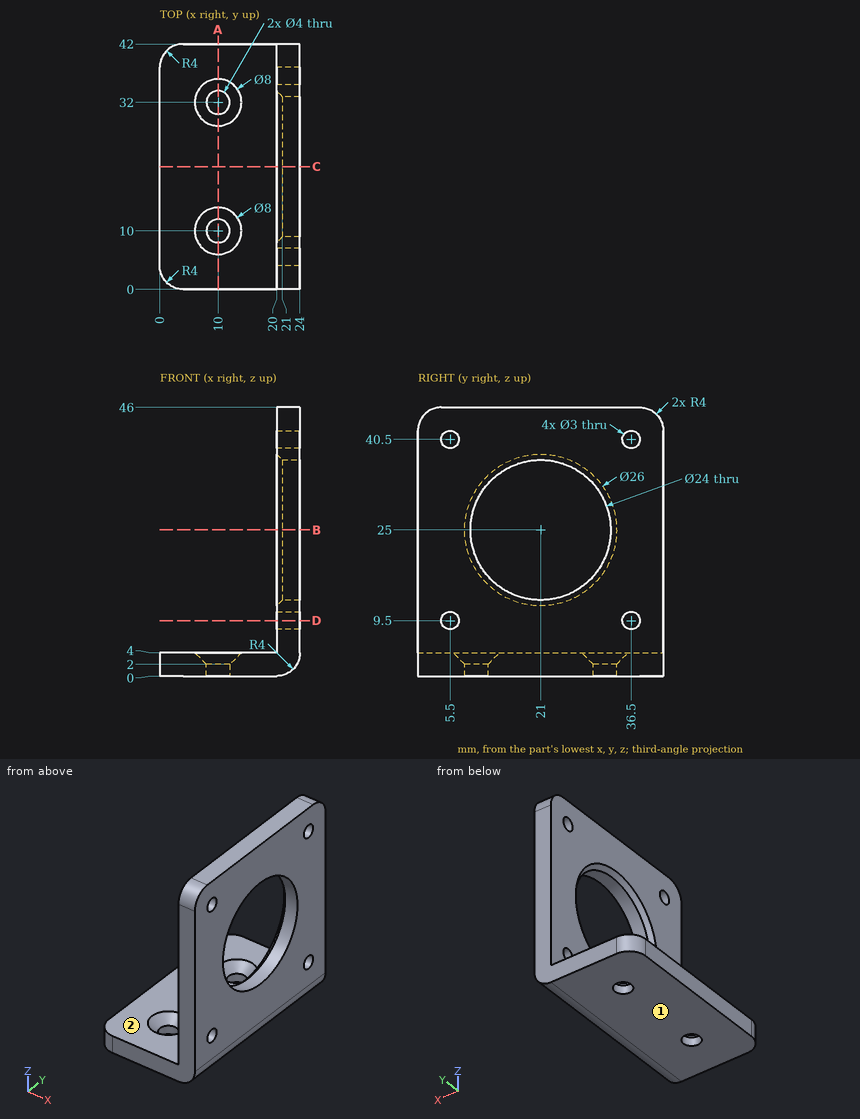
Study the drawing (mm; zero at the part's minimum x, y, z) and answer. A direction names the side the tool comes from. Round coordinates to 2 decimals unless told otherwise and drop trailing zeros. Write each loop counter-clockwise with the first axis right and the second up, starting at its lowest first coordinate (ties: lowest second). Pieces come first, ordered by that corner, then holes.
1) Straight lines are drawn through the part: line 1 (Y direction, x = 22, z = 9.5); line 2 (Y direction, x = 10, z = 1.45); line 3 (Y direction, x = 21.7, z = 25). For each, find the intervals that lie inside material, in ascending order.
2) A cutting plane is placed at B-B (z = 25). Give the vertices of the cut face in (x, y), plus the area to 3 significant figures.
3) Given pin 1 Ø4 at (y, z) = (5.5, 9.5) entering from -X; pin 2 Ø6 at (x, z) = (16, 16) entering from +Y; pin 3 Ø4 at (y, z) = (36.5, 9.5) entering from +X; pin 4 Ø5 at (x, y) = (8.5, 25.5) entering from +Z, each flat-ended and moving along its own axis, determine where each tip first touches the part or whether it passes through.
4) A tool of negligible diameter and unlimited length cuts with its end or side. For the marked faces 1 and 2, from which of +Z, -Z, +X, -X, +Y, -Y can it reach the whole face along a straight path? Write none if from no direction.
5) A cutting plane is placed at C-C (y = 21). Give the vertices of the cut face in (x, z).
6) A cutting plane is placed at D-D (z = 9.5). Give the vertices of the cut face in (x, y).
7) A cutting plane is placed at A-A (x = 10). Give the vertices of the cut face in (y, z), plus the area to 3 significant figures.
Completed:
1. line 1: y = 0 to 4, 7 to 35, 38 to 42
1. line 2: y = 0 to 8, 12 to 30, 34 to 42
1. line 3: y = 0 to 9, 33 to 42
2. outline: (20, 0) - (24, 0) - (24, 9) - (21, 9) - (20, 8) - close; (20, 34) - (21, 33) - (24, 33) - (24, 42) - (20, 42) - close
2. area: 71.0 mm2
3. pin 1: stops at x = 20
3. pin 2: passes through
3. pin 3: stops at x = 24
3. pin 4: stops at z = 4
4. face 1: -Z, +X, -X, +Y, -Y
4. face 2: +Z, -X, +Y, -Y
5. outline: (0, 0) - (20, 0) arc R4 ccw to (24, 4) - (24, 13) - (21, 13) - (20, 12) - (20, 4) - (0, 4) - close; (20, 38) - (21, 37) - (24, 37) - (24, 46) - (20, 46) - close
6. outline: (20, 0) - (24, 0) - (24, 4) - (20, 4) - close; (20, 7) - (24, 7) - (24, 35) - (20, 35) - close; (20, 38) - (24, 38) - (24, 42) - (20, 42) - close
7. outline: (0, 0) - (8, 0) - (8, 2) - (6, 4) - (0, 4) - close; (12, 0) - (30, 0) - (30, 2) - (28, 4) - (14, 4) - (12, 2) - close; (34, 0) - (42, 0) - (42, 4) - (36, 4) - (34, 2) - close
7. area: 128 mm2
